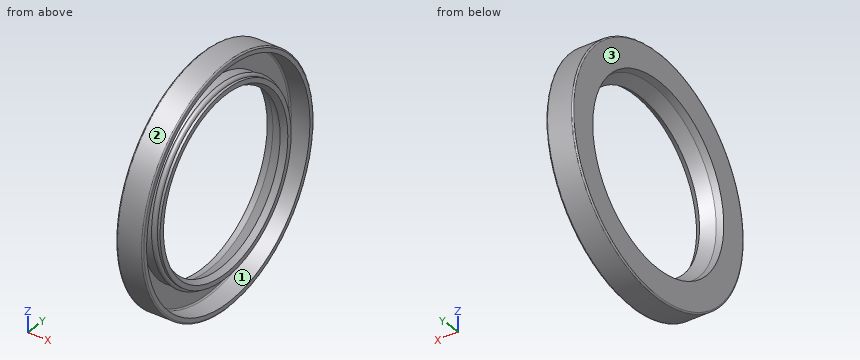
Autodesk Inventor part; units mm, degrees
ref_plane "YZ Plane" through (0, 0, 0) normal (1, 0, 0) x (0, 1, 0)
ref_plane "XZ Plane" through (0, 0, 0) normal (0, 1, 0) x (-1, 0, 0)
ref_plane "XY Plane" through (0, 0, 0) normal (0, 0, 1) x (1, 0, 0)
sketch "Skizze1" plane through (0, 0, 0) normal (0, 0, 1) x (1, 0, 0)
  circle A0 centre (7, 34.5) radius 0.65
  circle A1 centre (7, 34.5) radius 1
  line L0 (9, 32.75) -> (9, 34.5)
  line L1 (0, 45) -> (10, 45)
  line L2 (10, 45) -> (10, 43)
  line L3 (10, 43) -> (2.5, 43)
  line L4 (0, 0) -> (9.5856, 0)
  line L5 (0, 45) -> (0, 34.5)
  line L6 (0, 34.5) -> (2.5, 34)
  line L7 (2.5, 34) -> (7, 31.5)
  line L8 (7, 31.5) -> (9, 32.75)
  line L9 (7, 31.5) -> (0, 31.5) construction
  line L10 (0, 18) -> (0, -3)
  line L11 (-1.9171, 0) -> (11.5027, 0)
  line L12 (6, 34.5) -> (2.5, 35.2)
  line L13 (2.5, 35.2) -> (2.5, 43)
  line L14 (9, 34.5) -> (8, 34.5)
  dimension "d0" = 90
  dimension "d1" = 65.5
  dimension "d2" = 2
  dimension "d3" = 1.3
  dimension "d4" = 2
  dimension "d5" = 63
  dimension "d6" = 68
  dimension "d7" = 69
  dimension "d8" = 7
  dimension "d9" = 9
  dimension "d10" = 10
  dimension "d12" = 2.5
revolve "Körper" add sketch "Skizze1" angle 360 about axis through (0, 0, 0) along (1, 0, 0) contours L14 L0 L8 L7 L6 L5 L1 L2 L3 L13 L12 A1
revolve "Feder1" add sketch "Skizze1" angle 360 about axis through (0, 0, 0) along (1, 0, 0) contours A0 | A1
fillet "Rundung1" radius 0.5 3 edges at (10, -45, 0) (2.5, -43, 0) (0, -45, 0)
equation "\"d0\" = SD2"
equation "\"d1\" = ABDM"
equation "\"d3\" = SPDI"
equation "\"d4\" = SPDA"
equation "\"d5\" = NND"
equation "\"d6\" = TKDM"
equation "\"d7\" = HLDM"
equation "\"d8\" = SPDST"
equation "\"d9\" = SDI"
equation "\"d10\" = SWDT"
equation "\"d12\" = SD"
equation "\"d11\" = RR"
equation "\"SD2\" = 90"
equation "\"SWDT\" = 10"
equation "\"RR\" = 0.5"
equation "\"SD\" = 2.5"
equation "\"NND\" = 63"
equation "\"SPDA\" = 2"
equation "\"SPDI\" = 1.3"
equation "\"TKDM\" = 68"
equation "\"HLDM\" = 69"
equation "\"ABDM\" = 65.5"
equation "\"SDI\" = 9"
equation "\"SPDST\" = 7"
equation "\"LAB\" = 0.5"
properties part number "DIN 3760 - A - 63 x 90 x 10 - NBR" material "Gummi"
Build history of the part. All positions in model axes, mm. Face numbers are marked on the shaded views. Round coordinates to 2 decimals unless told otherwise and drop trailing zeros. Loops run counter-clockwise (first coordinate to the right, second up) from the corner with the lowest first, then second, coordinate; pieces in that order, holes last. Notation, with made-up numbers: (39, 89.5) -> (84, 89.5) arc R29 cw to (84, 123.5) -> close; hole circle Ø2 at (75.5, 30.25). An arc over 180 degrees is marked (long way). One line per item, written item: value. Start each with the question number.
Q1. Drop flat-ended pins along their axis: pin 1 Ø1 at (x, y) = (4.5, -36) entering from +Z; pin 2 Ø20.5 at (y, z) = (14.5, 12) entering from +X; pin 3 Ø1 at (x, z) = (7, 24.5) entering from +Y; pin 4 Ø3 at (x, z) = (8.5, -19) entering from +Y. Give the stop position or say it passes through.
Q2. Two-plate mould, pull along Z, no slides. Class the marked faces 1, 2 and 3: released by +Z, released by -Z, zero draft, split by the parting line, or undercut.
Q3. Cut at C-C on x = 4.75. List the corners of the cut face in (y, z).
Q4. Probe line 1 along Z through (x, y) = (7.25, 0); line 2 along Y through (x, z) = (6.5, 20.5); line 3 along Z through (x, y) = (7, 12). List the from-to ranges inside material, lowest first.
Computed:
1. pin 1: z = 27.65
1. pin 2: through
1. pin 3: y = 38.07
1. pin 4: y = 41.46
2. face 1: undercut
2. face 2: split by the parting line
2. face 3: zero draft
3. outline: circle Ø90 at (0, 0); circle Ø69.5 at (0, 0); hole circle Ø86 at (0, 0); hole circle Ø65.5 at (0, 0)
4. line 1: -45 to -43, -35.47 to -31.66, 31.66 to 35.47, 43 to 45
4. line 2: -40.06 to -37.8, -28.82 to -24.28, 24.28 to 28.82, 37.8 to 40.06
4. line 3: -43.37 to -41.29, -33.41 to -29.12, 29.12 to 33.41, 41.29 to 43.37
